Check sheet for the modelled part. Datum: model origin and axes. Units: mm. A direction names the side the tool comes from. Round coordinates to 2 decimals unless told otherwise and drop trailing zeros. Write each loop counter-clockwise with the first axis right and the second up, starting at its lowest first coordinate (ties: lowest second). Pieces come first, ordered by that corner, then holes.
Item 1: Release check for a two-part mould opening along Y. For faces 1 (the flat face through (4, -1.5, -1)), 2 (the flat face through (-4, 2.25, 1)), 3 (the cylindrical face through (2.5, 2.8, 0)) record: pulls with the +Y half, pulls with the -Y half, needs draft (parallel to the pull), parting line crosses it, or undercut.
Item 2: Section check C-C, the plane y = -1. Record the cut outline in (x, z).
Item 3: Material ranges on line 1 along Y through (x, z) = (-5, 1.55); line 2 along X through (y, z) = (-3.5, 0.05); line 3 along Z through (x, y) = (5, 0.4), recorded low to high.
Item 4: Set-up check for faces 4 (the cylindrical face through (2.5, -2.7, 0)), 5 (the flat face through (0, 0, -2)), 6 (the cylindrical face through (-2.5, 0, 0)): record each of +Z, -Z, +X, -X, +Y, -Y from which the full face is reachable in a straight line by a thin tool's end or side.
Item 5: Section check A-A, the plane x = 4.25. Record the cut outline in (y, z), plus the area to 3 significant figures.
Item 6: Section check B-B, the plane z = -1.05. Record the cut outline in (x, y).
Item 7: Depth check by flat-ended pin: pin 1 (1.5 mm diameter, centred on x = 5.5, z = -1.5, fed in from +Y); pin 2 (2 mm diameter, centred on x = -5, z = 0, fed in from +Y); pin 3 (2 mm diameter, centred on x = 4.5, z = -0.5, fed in from -Y); pin 4 (1.5 mm diameter, centred on y = -0.5, z = 1.5, fed in from -X). Enter the tip coordinate at first touch or a pass-through.
Item 8: Section check D-D, the plane x = -3.25. Record the cut outline in (y, z).
from build123d import *

# Parameters (mm, degrees)
CYLINDER001_R          = 2.5
CYLINDER001_DEPTH      = 2.5
CYLINDER001_ROLL_ANGLE = 90
CYLINDER002_R          = 2.5
CYLINDER002_DEPTH      = 2.5
CYLINDER002_ROLL_ANGLE = 90
CYLINDER_R             = 2.5
CYLINDER_DEPTH         = 4.5
CYLINDER_ROLL_ANGLE    = 90
SKETCH_R               = 1.25
PAD_DEPTH              = 4


with BuildPart() as cylinder001:
    # Cylinder001 → Cylinder001 (new body)
    with BuildSketch(Plane.XY):
        Circle(CYLINDER001_R)
    extrude(amount=CYLINDER001_DEPTH)


with BuildPart() as cylinder001_1:
    # Cylinder001 roll: moved
    add(cylinder001.part.rotate(Axis((0, 0, 0), (1, 0, 0)), CYLINDER001_ROLL_ANGLE))


with BuildPart() as cylinder001_2:
    # Cylinder001 placement: moved
    add(cylinder001_1.part.moved(Location((5, 4, 0))))


with BuildPart() as cylinder002:
    # Cylinder002 → Cylinder002 (new body)
    with BuildSketch(Plane.XY):
        Circle(CYLINDER002_R)
    extrude(amount=CYLINDER002_DEPTH)


with BuildPart() as cylinder002_1:
    # Cylinder002 roll: moved
    add(cylinder002.part.rotate(Axis((0, 0, 0), (1, 0, 0)), CYLINDER002_ROLL_ANGLE))


with BuildPart() as cylinder002_2:
    # Cylinder002 placement: moved
    add(cylinder002_1.part.moved(Location((5, -1.5, 0))))


with BuildPart() as axes_cutout:
    # Cylinder → Cylinder (new body)
    with BuildSketch(Plane.XY):
        Circle(CYLINDER_R)
    extrude(amount=CYLINDER_DEPTH)


with BuildPart() as axes_cutout_1:
    # Cylinder roll: moved
    add(axes_cutout.part.rotate(Axis((0, 0, 0), (1, 0, 0)), CYLINDER_ROLL_ANGLE))


with BuildPart() as axes_cutout_2:
    # Cylinder placement: moved
    add(axes_cutout_1.part.moved(Location((-5, 2.25, 0))))

    # Fusion: union Cylinder001, Cylinder002
    add(cylinder001_2.part)
    add(cylinder002_2.part)


with BuildPart() as track_shape:
    # Sketch → Pad (new body, symmetric)
    with BuildSketch(Plane.XZ):
        with BuildLine():
            Line((-5.1, 2), (5.1, 2))
            ThreePointArc((7, 0.1), (6.443503, 1.443503), (5.1, 2))
            Line((7, 0.1), (7, -0.1))
            ThreePointArc((5.1, -2), (6.443503, -1.443503), (7, -0.1))
            Line((5.1, -2), (-5.1, -2))
            ThreePointArc((-7, -0.1), (-6.443503, -1.443503), (-5.1, -2))
            Line((-7, -0.1), (-7, 0.1))
            ThreePointArc((-5.1, 2), (-6.443503, 1.443503), (-7, 0.1))
        make_face()
        with Locations((-5, 0)):
            Circle(SKETCH_R, mode=Mode.SUBTRACT)
        with Locations((5, 0)):
            Circle(SKETCH_R, mode=Mode.SUBTRACT)
    extrude(amount=PAD_DEPTH, both=True)

    # Cut: cut axes-cutout
    add(axes_cutout_2.part, mode=Mode.SUBTRACT)


solid = track_shape.part
Values found:
1. face 1: pulls with the -Y half
1. face 2: undercut
1. face 3: needs draft
2. outline: (-3.5, -2) - (5.1, -2) arc R1.9 ccw to (7, -0.1) - (7, 0.1) arc R1.9 ccw to (5.1, 2) - (-3.5, 2) arc R2.5 cw to start; hole circle Ø2.5 at (5, 0)
3. line 1: y = -4 to -2.25, 2.25 to 4
3. line 2: x = -7 to -6.25, -3.75 to 2.5
3. line 3: z = -2 to -1.25, 1.25 to 2
4. face 4: +X, -Y
4. face 5: -Z, +X, -X, +Y, -Y
4. face 6: -X
5. outline: (-1.5, -2) - (1.5, -2) - (1.5, -1) - (-1.5, -1) - close; (-1.5, 1) - (1.5, 1) - (1.5, 2) - (-1.5, 2) - close
5. area: 6.00 mm2
6. outline: (-6.75, -4) - (-5.68, -4) - (-5.68, -2.25) - (-6.75, -2.25) - close; (-6.75, 2.25) - (-5.68, 2.25) - (-5.68, 4) - (-6.75, 4) - close; (-4.32, -4) - (2.73, -4) - (2.73, -1.5) - (4.32, -1.5) - (4.32, 1.5) - (2.73, 1.5) - (2.73, 4) - (-4.32, 4) - (-4.32, 2.25) - (-2.73, 2.25) - (-2.73, -2.25) - (-4.32, -2.25) - close; (5.68, -1.5) - (6.75, -1.5) - (6.75, 1.5) - (5.68, 1.5) - close
7. pin 1: stops at y = 1.5
7. pin 2: passes through
7. pin 3: stops at y = -1.5
7. pin 4: stops at x = -3.5
8. outline: (-4, -2) - (4, -2) - (4, 2) - (-4, 2) - close; hole (-2.25, -1.79) - (2.25, -1.79) - (2.25, 1.79) - (-2.25, 1.79) - close
